Could you check a few things on this model? Use its own coordinates, in mm. A direction names the side the tool comes from. Round coordinates to 2 decimals unless told otherwise and drop trailing zeros. Loops run counter-clockwise (first coordinate to the right, second up) from the corner with the lowest first, then second, coordinate; pieces in that order, holes last. Notation, with made-up numbers: M 45.25,5.5 L 61.25,5.5 A18 cw 61.25,33.5 Z; hole C 0.5,47 d2. An arc over 180 degrees is marked long. One line per item, written item: value. Start each with the question number.
Q1. Please list where these lines run through material, in increasing order: line 1 along X through (y, z) = (8.25, 14.5); line 2 along X through (y, z) = (2, -26.5); line 3 along Z through (x, y) = (112.5, 0.5).
Q2. Which directions (+Z, -Z, +X, -X, +Y, -Y) give clear straight access to the entire face, cutting with the end or side of a thin tool? Please do faces 1 (the face through (2.437, 1.565, 5.792)), 2 (the face through (119.581, 1.565, -18.985)), 3 (the face through (-3, 9.525, -26)), 4 (the face through (111, 7, -135.738)), 5 (the face through (146.761, 7, -29)).
Q3. Imagine slicing it at C-C (z = -13). Please give me the cut outline in (x, y) (1 decimal).
Q4. I'm going to push flat-ended pins straight in: pin 1 Ø3.5 at (x, y) = (71, 2) entering from +Z; pin 2 Ø2.5 at (x, y) = (-3.5, 6) entering from -Z; pin 3 Ø2 at (y, z) = (4, -100) entering from -X. Where does each tip first touch, or does it pass through?
Q5. Imagine slicing it at B-B (x = 59). Please give me the cut outline in (y, z) (3 decimals), then the cut area to 3 significant figures.
Q6. Imagine slicing it at A-A (z = -81). Please give me the cut outline in (x, y) (3 decimals).
Q7. Imagine slicing it at D-D (y = 6.75). Give the number of separate pieces and of enclosed holes in the cut face, then the cut area to 3 significant figures.
from build123d import *

# Parameters (mm, degrees)
BOSS_EXTRUDE1_DEPTH = 3.175
SKETCH3_W           = 7.9375
SKETCH3_H           = 10.16
CUT_EXTRUDE1_DEPTH  = 3.175
SKETCH4_R           = 3.3909
BOSS_EXTRUDE2_DEPTH = 6.35
FILLET1_R           = 1.27
FILLET2_R           = 1.27
FILLET3_R           = 1.27
FILLET4_R           = 1.27


with BuildPart() as part:
    # Sketch1 → Boss-Extrude1 (new body)
    with BuildSketch(Plane(origin=(0, 0, 0), x_dir=(1, 0, 0), z_dir=(0, 1, 0))):
        with BuildLine():
            Line((0, 0), (0, 127.635))
            ThreePointArc((0, 127.635), (2.373196595, 133.364403405), (8.1026, 135.7376))
            Line((8.1026, 135.7376), (138.6586, 135.7376))
            ThreePointArc((138.6586, 135.7376), (144.388003405, 133.364403405), (146.7612, 127.635))
            Line((146.7612, 127.635), (146.7612, 0))
            ThreePointArc((146.7612, 0), (144.388003405, -5.729403405), (138.6586, -8.1026))
            Line((138.6586, -8.1026), (8.1026, -8.1026))
            ThreePointArc((8.1026, -8.1026), (2.373196595, -5.729403405), (0, 0))
        make_face()
        with BuildLine():
            Line((25.4, 104.418889077), (25.4, 23.216110923))
            ThreePointArc((25.4, 23.216110923), (27.133550294, 19.030950294), (31.318710923, 17.2974))
            Line((31.318710923, 17.2974), (115.442489077, 17.2974))
            ThreePointArc((115.442489077, 17.2974), (119.627649706, 19.030950294), (121.3612, 23.216110923))
            Line((121.3612, 23.216110923), (121.3612, 104.418889077))
            ThreePointArc((121.3612, 104.418889077), (119.627649706, 108.604049706), (115.442489077, 110.3376))
            Line((115.442489077, 110.3376), (31.318710923, 110.3376))
            ThreePointArc((31.318710923, 110.3376), (27.133550294, 108.604049706), (25.4, 104.418889077))
        make_face(mode=Mode.SUBTRACT)
    extrude(amount=BOSS_EXTRUDE1_DEPTH)

    # Sketch3 → Cut-Extrude1 (cut)
    with BuildSketch(Plane(origin=(0, 3.175, 0), x_dir=(1, 0, 0), z_dir=(0, 1, 0))):
        with Locations((7.14375, 114.7826)):
            Rectangle(SKETCH3_W, SKETCH3_H)
        with Locations((139.61745, 114.7826)):
            Rectangle(SKETCH3_W, SKETCH3_H)
        with Locations((139.61745, 12.8524)):
            Rectangle(SKETCH3_W, SKETCH3_H)
        with Locations((7.14375, 12.8524)):
            Rectangle(SKETCH3_W, SKETCH3_H)
    extrude(amount=-CUT_EXTRUDE1_DEPTH, mode=Mode.SUBTRACT)

    # Sketch4 → Boss-Extrude2 (add, symmetric)
    # profile 1 of 8: a face of its own
    with BuildSketch(Plane(origin=(0, 3.175, 0), x_dir=(1, 0, 0), z_dir=(0, 1, 0))):
        with BuildLine():
            Line((28.9306, 135.7376), (41.6306, 135.7376))
            Line((41.6306, 135.7376), (41.6306, 142.0876))
            ThreePointArc((41.6306, 142.0876), (35.2806, 148.4376), (28.9306, 142.0876))
            Line((28.9306, 142.0876), (28.9306, 135.7376))
        make_face()
        with Locations(Location((35.2806, 142.0876, 0), (0, 0, 270))):
            Circle(SKETCH4_R, mode=Mode.SUBTRACT)
    # profile 2 of 8: a face of its own
    with BuildSketch(Plane(origin=(0, 3.175, 0), x_dir=(1, 0, 0), z_dir=(0, 1, 0))):
        with BuildLine():
            Line((41.6306, -8.1026), (41.6306, -14.4526))
            ThreePointArc((41.6306, -14.4526), (34.504736276, -20.755022985), (29.120195124, -12.912498781))
            Line((29.120195124, -12.912498781), (28.9306, -8.1026))
            Line((28.9306, -8.1026), (41.6306, -8.1026))
        make_face()
        with Locations(Location((35.2806, -14.4526, 0), (0, 0, 270))):
            Circle(SKETCH4_R, mode=Mode.SUBTRACT)
    # profile 3 of 8: a face of its own
    with BuildSketch(Plane(origin=(0, 3.175, 0), x_dir=(1, 0, 0), z_dir=(0, 1, 0))):
        with BuildLine():
            Line((117.8306, -8.1026), (117.641004876, -12.912498781))
            ThreePointArc((117.641004876, -12.912498781), (112.256463724, -20.755022985), (105.1306, -14.4526))
            Line((105.1306, -14.4526), (105.1306, -8.1026))
            Line((105.1306, -8.1026), (117.8306, -8.1026))
        make_face()
        with Locations(Location((111.4806, -14.4526, 0), (0, 0, 270))):
            Circle(SKETCH4_R, mode=Mode.SUBTRACT)
    # profile 4 of 8: a face of its own
    with BuildSketch(Plane(origin=(0, 3.175, 0), x_dir=(1, 0, 0), z_dir=(0, 1, 0))):
        with BuildLine():
            Line((117.8306, 135.7376), (117.8306, 142.0876))
            ThreePointArc((117.8306, 142.0876), (111.4806, 148.4376), (105.1306, 142.0876))
            Line((105.1306, 142.0876), (105.1306, 135.7376))
            Line((105.1306, 135.7376), (117.8306, 135.7376))
        make_face()
        with Locations(Location((111.4806, 142.0876, 0), (0, 0, 90))):
            Circle(SKETCH4_R, mode=Mode.SUBTRACT)
    # profile 5 of 8: a face of its own
    with BuildSketch(Plane(origin=(0, 3.175, 0), x_dir=(1, 0, 0), z_dir=(0, 1, 0))):
        with BuildLine():
            Line((146.7612, 92.362412849), (146.7612, 105.062412849))
            Line((146.7612, 105.062412849), (153.1112, 105.062412849))
            ThreePointArc((153.1112, 105.062412849), (159.4612, 98.712412849), (153.1112, 92.362412849))
            Line((153.1112, 92.362412849), (146.7612, 92.362412849))
        make_face()
        with Locations(Location((153.1112, 98.712412849, 0), (0, 0, 270))):
            Circle(SKETCH4_R, mode=Mode.SUBTRACT)
    # profile 6 of 8: a face of its own
    with BuildSketch(Plane(origin=(0, 3.175, 0), x_dir=(1, 0, 0), z_dir=(0, 1, 0))):
        with BuildLine():
            Line((146.7612, 22.572587151), (153.1112, 22.572587151))
            ThreePointArc((153.1112, 22.572587151), (159.4612, 28.922587151), (153.1112, 35.272587151))
            Line((153.1112, 35.272587151), (146.7612, 35.272587151))
            Line((146.7612, 35.272587151), (146.7612, 22.572587151))
        make_face()
        with Locations(Location((153.1112, 28.922587151, 0), (0, 0, 90))):
            Circle(SKETCH4_R, mode=Mode.SUBTRACT)
    # profile 7 of 8: a face of its own
    with BuildSketch(Plane(origin=(0, 3.175, 0), x_dir=(1, 0, 0), z_dir=(0, 1, 0))):
        with BuildLine():
            Line((-6.35, 35.272587151), (0, 35.272587151))
            Line((0, 35.272587151), (0, 22.572587151))
            Line((0, 22.572587151), (-6.35, 22.572587151))
            ThreePointArc((-6.35, 22.572587151), (-12.7, 28.922587151), (-6.35, 35.272587151))
        make_face()
        with Locations(Location((-6.35, 28.922587151, 0), (0, 0, 270))):
            Circle(SKETCH4_R, mode=Mode.SUBTRACT)
    # profile 8 of 8: a face of its own
    with BuildSketch(Plane(origin=(0, 3.175, 0), x_dir=(1, 0, 0), z_dir=(0, 1, 0))):
        with BuildLine():
            Line((0, 92.362412849), (0, 105.062412849))
            Line((0, 105.062412849), (-6.35, 105.062412849))
            ThreePointArc((-6.35, 105.062412849), (-12.7, 98.712412849), (-6.35, 92.362412849))
            Line((-6.35, 92.362412849), (0, 92.362412849))
        make_face()
        with Locations(Location((-6.35, 98.712412849, 0), (0, 0, 270))):
            Circle(SKETCH4_R, mode=Mode.SUBTRACT)
    extrude(amount=BOSS_EXTRUDE2_DEPTH, both=True)

    # Fillet1
    fillet1_edges = [part.edges().sort_by_distance(p)[0] for p in [
        (28.9306, 1.5875, 8.1026),
        (41.6306, 1.5875, 8.1026),
    ]]
    fillet(fillet1_edges, radius=FILLET1_R)

    # Fillet2
    fillet2_edges = [part.edges().sort_by_distance(p)[0] for p in [
        (35.2806, 0, 8.1026),
        (35.2806, 3.175, 8.1026),
    ]]
    fillet(fillet2_edges, radius=FILLET2_R)

    # Fillet3
    fillet3_edges = [part.edges().sort_by_distance(p)[0] for p in [
        (0, 0, -28.922587151),
        (0, 3.175, -28.922587151),
        (111.4806, 3.175, 8.1026),
        (111.4806, 0, 8.1026),
        (146.7612, 0, -28.922587151),
        (146.7612, 3.175, -28.922587151),
        (146.7612, 0, -98.712412849),
        (146.7612, 3.175, -98.712412849),
        (111.4806, 0, -135.7376),
        (111.4806, 3.175, -135.7376),
        (35.2806, 3.175, -135.7376),
        (35.2806, 0, -135.7376),
        (0, 0, -98.712412849),
        (0, 3.175, -98.712412849),
    ]]
    fillet(fillet3_edges, radius=FILLET3_R)

    # Fillet4
    fillet4_edges = [part.edges().sort_by_distance(p)[0] for p in [
        (0, 1.5875, -35.272587151),
        (0, 1.5875, -22.572587151),
        (117.8306, 1.5875, 8.1026),
        (105.1306, 1.5875, 8.1026),
        (146.7612, 1.5875, -35.272587151),
        (146.7612, 1.5875, -22.572587151),
        (146.7612, 1.5875, -105.062412849),
        (146.7612, 1.5875, -92.362412849),
        (105.1306, 1.5875, -135.7376),
        (117.8306, 1.5875, -135.7376),
        (28.9306, 1.5875, -135.7376),
        (41.6306, 1.5875, -135.7376),
        (0, 1.5875, -92.362412849),
        (0, 1.5875, -105.062412849),
    ]]
    fillet(fillet4_edges, radius=FILLET4_R)


solid = part.part
Report:
1. line 1: x = 28.93 to 31.89, 38.67 to 41.63, 105.13 to 108.09, 114.87 to 117.83
1. line 2: x = -12.22 to -8.72, -3.98 to 25.4, 121.36 to 150.74, 155.48 to 158.98
1. line 3: z = -148.36 to -145.32, -138.85 to -110.34, -17.3 to 11.22, 17.69 to 20.72
2. face 1: +Z, -X, +Y, -Y
2. face 2: +Y, -Y
2. face 3: +Z, -Z, +X, -X, +Y
2. face 4: +X, -X, +Y
2. face 5: +Z, -Z, +Y
3. outline: M 0,0 L 3.2,0 L 3.2,3.2 L 0,3.2 Z; M 11.1,0 L 135.6,0 L 135.6,3.2 L 11.1,3.2 Z; M 143.6,0 L 146.8,0 L 146.8,3.2 L 143.6,3.2 Z
4. pin 1: stops at z = 8.1
4. pin 2: stops at z = -105.06
4. pin 3: stops at x = -12.69
5. outline: M 0,-135.738 L 3.175,-135.738 L 3.175,-110.338 L 0,-110.338 Z; M 0,-17.297 L 3.175,-17.297 L 3.175,8.103 L 0,8.103 Z
5. area: 161 mm²
6. outline: M 0,0 L 25.4,0 L 25.4,3.175 L 0,3.175 Z; M 121.361,0 L 146.761,0 L 146.761,3.175 L 121.361,3.175 Z
7. separate pieces: 8
7. enclosed holes: 8
7. area: 862 mm²
